Work out the finished part from the listing and answer in its coordinate system (mm). A direction names the side the tool comes from. Coordinates: 2 decimals unless noted, no trailing zeros. Order: outer loops, then holes, each group sorted by start corner. A loop starts at its lowest first (then second) coordinate and runs counter-clockwise, first axis right, second up.
1. The part is cut by section B-B, the plane z = 307.5. Give the vertices of the cut face in (x, y).
2. Determine the mould class of faces 1 (the flat face through (46, -3, 330)), 2 (the cylindrical face through (-11.923, -53.692, 177.62)), 3 (the flat face through (0, -43, 0)) for opening direction X: +X half, -X half, draft (parallel to the pull), parting line (faces both ways), or undercut.
3. The part is cut by section A-A, the plane x = -22.5. Give the vertices of the cut face in (y, z).
4. A tool of negligible diameter and unlimited length cuts with its end or side. For faces 4 (the cylindrical face through (-50.076, 15.77, 4.93)), 5 (the flat face through (0, 44, 20)), 6 (the cylindrical face through (0.1, 42.5, 9.9)), from which of +Z, -Z, +X, -X, +Y, -Y can it reach the whole face along a straight path? Write none if from no direction.
5. The part is cut by section C-C, the plane x = 38. Give the vertices of the cut face in (y, z) (3 decimals).
6. Find the intervals of material crossed by probe 1 along X at (y, z) = (2.5, 298.5); probe 2 along X at (y, z) = (1, 118.5); probe 3 along Y at (x, z) = (0, 83), in increasing order.
7. Flat-ended cylindrical pins translate along their axes: pin 1 Ø3 at (x, y) = (1.5, -47.5) entering from -Z; pin 2 Ø2 at (x, z) = (0.5, 330.5) entering from +Y; pin 3 Ø2 at (y, z) = (41.5, 187) entering from +X; pin 4 Ø12 at (x, z) = (-18.5, 129) entering from -Y. Find the tip coordinate at first contact, or state that the pin passes through.
```python
from build123d import *

# Parameters (mm, degrees)
SKETCH_2_R          = 55
SKETCH_2_R_2        = 50
EXTRUDE_1_DEPTH     = 350
SKETCH_1_R          = 55
SKETCH_1_R_2        = 1.5
EXTRUDE_2_DEPTH     = 20
CUT_EXTRUDE_1_DEPTH = 2
SKETCH_4_R          = 55
SKETCH_4_R_2        = 52.5
CUT_EXTRUDE_2_DEPTH = 10


with BuildPart() as part:
    # 草图2 → 凸台-拉伸1 (new body)
    with BuildSketch(Plane.XY):
        Circle(SKETCH_2_R)
        Circle(SKETCH_2_R_2, mode=Mode.SUBTRACT)
    extrude(amount=EXTRUDE_1_DEPTH)

    # 草图1 → 凸台-拉伸2 (add)
    with BuildSketch(Plane.XY):
        Circle(SKETCH_1_R)
        with Locations((0, -47)):
            Circle(SKETCH_1_R_2, mode=Mode.SUBTRACT)
        with Locations((47, 0)):
            Circle(SKETCH_1_R_2, mode=Mode.SUBTRACT)
        with Locations((0, 47)):
            Circle(SKETCH_1_R_2, mode=Mode.SUBTRACT)
        with Locations((-47, 0)):
            Circle(SKETCH_1_R_2, mode=Mode.SUBTRACT)
        with BuildLine():
            Line((-6.670179488, -49.553089768), (-3.897114317, -44.75))
            ThreePointArc((-3.897114317, -44.75), (0, -42.5), (3.897114317, -44.75))
            Line((3.897114317, -44.75), (6.670179488, -49.553089768))
            ThreePointArc((6.670179488, -49.553089768), (35.355339059, -35.355339059), (49.553089768, -6.670179488))
            Line((49.553089768, -6.670179488), (44.75, -3.897114317))
            ThreePointArc((44.75, -3.897114317), (42.5, 0), (44.75, 3.897114317))
            Line((44.75, 3.897114317), (49.553089768, 6.670179488))
            ThreePointArc((49.553089768, 6.670179488), (35.355339059, 35.355339059), (6.670179488, 49.553089768))
            Line((6.670179488, 49.553089768), (3.897114317, 44.75))
            ThreePointArc((3.897114317, 44.75), (0, 42.5), (-3.897114317, 44.75))
            Line((-3.897114317, 44.75), (-6.670179488, 49.553089768))
            ThreePointArc((-6.670179488, 49.553089768), (-35.355339059, 35.355339059), (-49.553089768, 6.670179488))
            Line((-49.553089768, 6.670179488), (-44.75, 3.897114317))
            ThreePointArc((-44.75, 3.897114317), (-42.5, 0), (-44.75, -3.897114317))
            Line((-44.75, -3.897114317), (-49.553089768, -6.670179488))
            ThreePointArc((-49.553089768, -6.670179488), (-35.355339059, -35.355339059), (-6.670179488, -49.553089768))
        make_face(mode=Mode.SUBTRACT)
    extrude_2 = extrude(amount=EXTRUDE_2_DEPTH)

    # 草图3 → 切除-拉伸1 (cut)
    with BuildSketch(Plane.XY.offset(20)):
        Polygon((-1.58771324, 44.25), (1.58771324, 44.25), (3.175426481, 47), (1.58771324, 49.75), (-1.58771324, 49.75), (-3.175426481, 47), align=None)
        Polygon((-44.25, -1.58771324), (-44.25, 1.58771324), (-47, 3.175426481), (-49.75, 1.58771324), (-49.75, -1.58771324), (-47, -3.175426481), align=None)
        Polygon((44.25, 1.58771324), (44.25, -1.58771324), (47, -3.175426481), (49.75, -1.58771324), (49.75, 1.58771324), (47, 3.175426481), align=None)
        Polygon((1.58771324, -44.25), (-1.58771324, -44.25), (-3.175426481, -47), (-1.58771324, -49.75), (1.58771324, -49.75), (3.175426481, -47), align=None)
    cut_extrude_1 = extrude(amount=-CUT_EXTRUDE_1_DEPTH, mode=Mode.SUBTRACT)

    # 镜向1: 凸台-拉伸2, 切除-拉伸1 across plane
    add(extrude_2.mirror(Plane(origin=(0, 0, 175), x_dir=(1, 0, 0), z_dir=(0, 0, -1))))
    add(cut_extrude_1.mirror(Plane(origin=(0, 0, 175), x_dir=(1, 0, 0), z_dir=(0, 0, -1))), mode=Mode.SUBTRACT)

    # 草图4 → 切除-拉伸2 (cut)
    with BuildSketch(Plane(origin=(0, 0, 0), x_dir=(-1, 0, 0), z_dir=(0, 0, -1))):
        Circle(SKETCH_4_R)
        Circle(SKETCH_4_R_2, mode=Mode.SUBTRACT)
    extrude(amount=-CUT_EXTRUDE_2_DEPTH, mode=Mode.SUBTRACT)


solid = part.part
```
Geometry says:
1. outline: circle Ø110 at (0, 0); hole circle Ø100 at (0, 0)
2. face 1: undercut
2. face 2: parting line
2. face 3: draft
3. outline: (-50.19, 10) - (-47.43, 10) - (-47.43, 0) - (-44.65, 0) - (-44.65, 350) - (-50.19, 350) - close; (44.65, 0) - (47.43, 0) - (47.43, 10) - (50.19, 10) - (50.19, 350) - (44.65, 350) - close
4. face 4: -Z
4. face 5: none
4. face 6: +Z, -Z
5. outline: (-39.762, 10) - (-36.225, 10) - (-36.225, 0) - (-32.496, 0) - (-32.496, 350) - (-39.762, 350) - close; (32.496, 0) - (36.225, 0) - (36.225, 10) - (39.762, 10) - (39.762, 350) - (32.496, 350) - close
6. probe 1: x = -54.94 to -49.94, 49.94 to 54.94
6. probe 2: x = -54.99 to -49.99, 49.99 to 54.99
6. probe 3: y = -55 to -50, 50 to 55
7. pin 1: stops at z = 0
7. pin 2: stops at y = 55
7. pin 3: stops at x = 37.21
7. pin 4: stops at y = -53.56
